from build123d import *

# Parameters (mm, degrees)
BOSS_EXTRUDE1_DEPTH = 9.525
SKETCH2_R           = 1.5875
CUT_EXTRUDE1_DEPTH  = 19.814239953


with BuildPart() as part:
    # Sketch1 → Boss-Extrude1 (new body)
    with BuildSketch(Plane(origin=(0, 0, 0), x_dir=(0, 0, -1), z_dir=(1, 0, 0))):
        with BuildLine():
            Line((-6.5, 0), (-13.5, 0))
            Line((-13.5, 0), (-13.5, 9))
            Line((-13.5, 9), (13.5, 9))
            Line((13.5, 9), (13.5, 0))
            Line((13.5, 0), (6.5, 0))
            ThreePointArc((6.5, 0), (0, 6.5), (-6.5, 0))
        make_face()
    extrude(amount=BOSS_EXTRUDE1_DEPTH)

    # Sketch2 → Cut-Extrude1 (cut, through all)
    with BuildSketch(Plane(origin=(0, 9, 0), x_dir=(1, 0, 0), z_dir=(0, 1, 0))):
        with Locations(Location((4.7625, -10.75, 0), (0, 0, 270))):
            Circle(SKETCH2_R)
        with Locations(Location((4.7625, 10.75, 0), (0, 0, 270))):
            Circle(SKETCH2_R)
    extrude(amount=-CUT_EXTRUDE1_DEPTH, mode=Mode.SUBTRACT)


solid = part.part
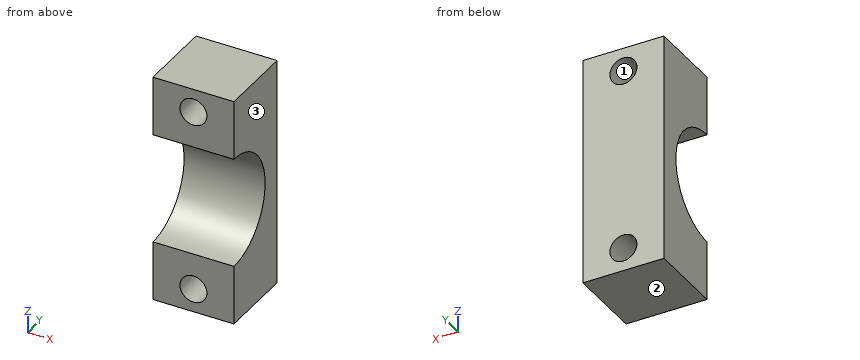
The model under review builds one solid part; all positions refer to its coordinate system, in mm. Face numbers are marked on the shaded views. Round coordinates to 2 decimals unless told otherwise and drop trailing zeros. Order: outer loops, then holes, each group sorted by start corner. A loop starts at its lowest first (then second) coordinate and runs counter-clockwise, first axis right, second up. Notation, with made-up numbers: (-4, -10.75) - (7, -10.75) arc R27 ccw to (7, 14.25) - close; hole circle Ø7 at (65.25, 51.25). An arc over 180 degrees is marked (long way). Use one line per item in the form item = value.
Q1. Mouldability with a two-part tool opening along Z and no side actions: class the marked faces 1, 2 and 3 as pulls with the +Z half, pulls with the -Z half, needs draft (parallel to the pull), parting line crosses it, or undercut.
Response values:
face_1 = undercut
face_2 = pulls with the -Z half
face_3 = needs draft
Q2. Add section C-C on x = 4. Give the boundary of the cut face in (y, z).
Response values:
outline = (0, -13.5) - (9, -13.5) - (9, -12.14) - (0, -12.14) - close; (0, -9.36) - (9, -9.36) - (9, 9.36) - (0, 9.36) - (0, 6.5) arc R6.5 cw to (0, -6.5) - close; (0, 12.14) - (9, 12.14) - (9, 13.5) - (0, 13.5) - close
Q3. Add section A-A on z = 10.75. Give the boundary of the cut face in (x, y) (3 decimals), then the cut area to 4 significant figures.
Response values:
outline = (0, 0) - (3.175, 0) - (3.175, 9) - (0, 9) - close; (6.35, 0) - (9.525, 0) - (9.525, 9) - (6.35, 9) - close
area = 57.15 mm^2
Q4. Add section B-B on y = 4.5. Give the number of separate pieces and of enclosed holes in the cut face, then the cut area to 3 significant figures.
Response values:
separate_pieces = 2
enclosed_holes = 2
area = 152 mm^2
Q5. To check wall thickness, follow line 1 (X direction, y = 5.25, z = -10.75) (3 decimals); line 2 (Z direction, x = 3.5, y = 2); line 3 (Z direction, x = 5.25, y = 2.5). State the ranges of each line that lie inside material, in increasing order.
Response values:
line_1 = 0 to 3.175, 6.35 to 9.525
line_2 = -13.5 to -11.71, -9.79 to -6.18, 6.18 to 9.79, 11.71 to 13.5
line_3 = -13.5 to -12.26, -9.24 to -6, 6 to 9.24, 12.26 to 13.5
Q6. Clearance check with a flat-ended pin moving along its axis: P1, Ø4, axis at x = 3, z = -6, coming from the -Y side. State where the tip first meets the part, or that it passes through.
Response values:
P1 = 0
